Design review of the part built by this model. Coordinates are the model's own, in mm. Face numbers are marked on the shaded views. A direction names the side the tool comes from. Coordinates: 2 decimals unless noted, no trailing zeros. Order: outer loops, then holes, each group sorted by start corner. A loop starts at its lowest first (then second) coordinate and runs counter-clockwise, first axis right, second up. Notation, with made-up numbers: M 47.5,77 L 100.5,77 A19 ccw 100.5,113 Z; hole C 83,87 d10. An arc over 180 degrees is marked long. Answer as a JSON object with one key per item and string values.
from build123d import *

# Parameters (mm, degrees)
BOSS_EXTRUDE1_DEPTH         = 3
FILLET1_R                   = 10
M3_TAPPED_HOLE1_D           = 2.5
M3_TAPPED_HOLE1_DEPTH       = 5
M3_TAPPED_HOLE1_CSINK_D     = 3.05
M3_TAPPED_HOLE1_CSINK_ANGLE = 90
M3_TAPPED_HOLE1_TIP         = 0.751075774
CUT_EXTRUDE1_DEPTH          = 6.5000001
SKETCH8_R                   = 1
CUT_EXTRUDE2_DEPTH          = 4
CUT_EXTRUDE2_DEPTH_BACK     = 4
CHAMFER1_SIZE               = 0.5


with BuildPart() as part:
    # Sketch1 → Boss-Extrude1 (new body, symmetric)
    with BuildSketch(Plane(origin=(0, 0, 0), x_dir=(1, 0, 0), z_dir=(0, 1, 0))):
        with BuildLine():
            Line((-2.5, -3.122498999), (-2.5, -18))
            Line((-2.5, -18), (2.5, -18))
            Line((2.5, -18), (2.5, -3.122498999))
            ThreePointArc((2.5, -3.122498999), (0, 4), (-2.5, -3.122498999))
        make_face()
    extrude(amount=BOSS_EXTRUDE1_DEPTH, both=True)

    # Fillet1
    fillet1_edges = [part.edges().sort_by_distance(p)[0] for p in [
        (-2.5, 0, 3.122498999),
        (2.5, 0, 3.122498999),
    ]]
    fillet(fillet1_edges, radius=FILLET1_R)

    # Sweep1: sweep along a path in Sketch3
    with BuildLine(Plane(origin=(0, 3, 0), x_dir=(1, 0, 0), z_dir=(0, 1, 0))) as sweep1_path:
        Line((2.5, -18), (2.5, -6.304760106))
        ThreePointArc((2.5, -6.304760106), (2.771543949, -3.990209857), (3.571428571, -1.80136003))
        ThreePointArc((3.571428571, -1.80136003), (0, 4), (-3.571428571, -1.80136003))
        ThreePointArc((-3.571428571, -1.80136003), (-2.771543949, -3.990209857), (-2.5, -6.304760106))
        Line((-2.5, -6.304760106), (-2.5, -18))
    # Sketch2 → Sweep1 (sweep)
    with BuildSketch(Plane.XY.offset(18)):
        with BuildLine():
            Line((2.5, 3), (2.5, -3))
            ThreePointArc((2.5, -3), (4, 0), (2.5, 3))
        make_face()
    sweep(path=sweep1_path.line)

    # M3 Tapped Hole1
    with Locations(Plane.XY.offset(18)):
        with Locations((0, 0)):
            CounterSinkHole(M3_TAPPED_HOLE1_D / 2, M3_TAPPED_HOLE1_CSINK_D / 2, depth=M3_TAPPED_HOLE1_DEPTH, counter_sink_angle=M3_TAPPED_HOLE1_CSINK_ANGLE)
            with Locations((0, 0, -(M3_TAPPED_HOLE1_DEPTH + M3_TAPPED_HOLE1_TIP / 2))):  # 118° drill point
                Cone(0, M3_TAPPED_HOLE1_D / 2, M3_TAPPED_HOLE1_TIP, mode=Mode.SUBTRACT)

    # Sketch6 → Cut-Extrude1 (cut, symmetric)
    with BuildSketch(Plane(origin=(0, 0, 0), x_dir=(0, 0, -1), z_dir=(1, 0, 0))):
        Polygon((-9, 3), (-8.5, 2.5), (11, 2.5), (11, 3), align=None)
    cut_extrude1 = extrude(amount=CUT_EXTRUDE1_DEPTH, both=True, mode=Mode.SUBTRACT)

    # Mirror1: Cut-Extrude1 across plane
    add(cut_extrude1.mirror(Plane.ZX), mode=Mode.SUBTRACT)

    # Sketch7 → Cut-Revolve1 (revolve, cut)
    with BuildSketch(Plane(origin=(0, 0, 0), x_dir=(0, 0, -1), z_dir=(1, 0, 0))):
        with BuildLine():
            Line((0, 3), (0, -3))
            Line((0, -3), (2.75, -3))
            Line((2.75, -3), (2.75, -1.198957881))
            ThreePointArc((2.75, -1.198957881), (3, 0), (2.75, 1.198957881))
            Line((2.75, 1.198957881), (2.75, 3))
            Line((2.75, 3), (0, 3))
        make_face()
    revolve(axis=Axis((0, 6.277574948, 0), (0, -1, 0)), mode=Mode.SUBTRACT)

    # Sketch8 → Cut-Extrude2 (cut, two sides)
    with BuildSketch(Plane(origin=(0, 0, 0), x_dir=(1, 0, 0), z_dir=(0, 1, 0))) as cut_extrude2_sk:
        with Locations((0, -7)):
            Circle(SKETCH8_R)
    extrude(amount=CUT_EXTRUDE2_DEPTH, mode=Mode.SUBTRACT)
    extrude(cut_extrude2_sk.sketch, amount=-CUT_EXTRUDE2_DEPTH_BACK, mode=Mode.SUBTRACT)

    # Chamfer1
    chamfer1_edges = [part.edges().sort_by_distance(p)[0] for p in [
        (0, 2.5, 2.75),
        (0, -2.5, 2.75),
    ]]
    chamfer(chamfer1_edges, length=CHAMFER1_SIZE)


solid = part.part
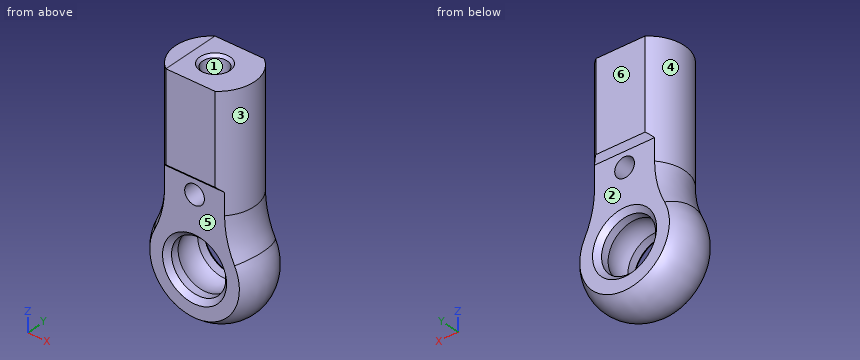
1) Tool access review of the marked faces 5 and 6: name each direction out of +Z, -Z, +X, -X, +Y, -Y from which nothing blocks a thin tool from reaching the whole face with its end or side.
Taken from the geometry:
{"face 5": "-Z, +X, -X, -Y", "face 6": "+Z, -Z, +X, -X, +Y"}
2) Add section C-C (z = 12.75). State the section outline as (x, y) points.
Taken from the geometry:
{"outline": "M -2.5,-3 L 2.5,-3 A3.75 ccw 2.5,3 L -2.5,3 A3.75 ccw Z; hole C 0,0 d1.67"}
3) Add section A-A (z = 7). State the section outline as (x, y) points, and give its area (3 significant figures).
Taken from the geometry:
{"outline": "M -3.05,-2.5 L -1,-2.5 L -1,2.5 L -3.05,2.5 A3.75 ccw Z; M 1,-2.5 L 3.05,-2.5 A3.75 ccw 3.05,2.5 L 1,2.5 Z", "area": "27.0 mm2"}
4) Mouldability with a two-part tool opening along X and no side actions: class the marked faces 1, 2, 3 and 4 as released by +X, released by -X, zero draft, split by the parting line, or undercut.
Taken from the geometry:
{"face 1": "undercut", "face 2": "zero draft", "face 3": "released by +X", "face 4": "released by -X"}
5) Insertion check: pin 1 Ø1.8 at (x, z) = (0, 7) entering from -Y; pin 2 Ø2 at (x, y) = (0, 0) entering from +Z; pin 3 Ø1 at (x, z) = (1.5, 3) entering from -Y; pin 4 Ø1.5 at (x, z) = (-3.5, 9.5) entering from -Y. Each pin has a flat end and moves straight along its axis. Give the tip position at first contact, or say it passes through.
Taken from the geometry:
{"pin 1": "passes through", "pin 2": "stops at z = 12.85", "pin 3": "stops at y = -2.5", "pin 4": "stops at y = -2.8"}
6) Add section B-B (y = -0.5). Count the separate pieces of the cut face and the enclosed holes in it, and give its area (3 significant figures).
Taken from the geometry:
{"separate pieces": "1", "enclosed holes": "2", "area": "156 mm2"}
7) To check wall thickness, follow L1, parallel to Y at x = 0, z = 14; L2, parallel to Z at x = 0, y = -1.6; L3, parallel to Z at x = 0, y = -1. State the ranges of each line that lie inside material, in increasing order.
Taken from the geometry:
{"L1": "y = -3 to -1.25, 1.25 to 3", "L2": "z = -5.14 to -2.75, 2.75 to 6, 8 to 18", "L3": "z = -5.36 to -2.83, 2.83 to 6, 8 to 12.85"}
